```python
from build123d import *

# Parameters (mm, degrees)
SKETCH2_W                        = 127
SKETCH2_H                        = 127
HOUSING_DEPTH                    = 39.5
SKETCH3_R                        = 19.05
CUT_EXTRUDE1_DEPTH               = 40.5
SKETCH4_OUTSIDE_W                = 165.78
SKETCH4_OUTSIDE_H                = 165.78
SKETCH4_OUTSIDE_R                = 45.974
CUT_EXTRUDE2_DEPTH               = 4.698
MOUNTING_POCKETS_DEPTH           = 24.384
ENG_METRIC_SLOT_VERTICAL_REACH   = 129
ENG_METRIC_SLOT_HORIZONTAL_DEPTH = 40.5
FILLET3_R                        = 0.508
F_10_32_TAPPED_HOLE1_D           = 4.0386
F_10_32_TAPPED_HOLE1_DEPTH       = 12.02944
F_10_32_TAPPED_HOLE1_TIP         = 1.213317848
SKETCH219_R                      = 53.086
EXTRUDE2_DEPTH                   = 10.414
SKETCH222_R                      = 53.086
SKETCH222_R_2                    = 46.99
CUT_EXTRUDE6_DEPTH               = 6.35
LPATTERN14_COUNT                 = 3
LPATTERN14_PITCH                 = 25.4
LPATTERN14_COUNT_DIR2            = 3
LPATTERN14_PITCH_DIR2            = 25.4
M6X1_0_TAPPED_HOLE1_D            = 5
M6X1_0_TAPPED_HOLE1_DEPTH        = 8
M6X1_0_TAPPED_HOLE1_CBORE_D      = 6
M6X1_0_TAPPED_HOLE1_CBORE_DEPTH  = 6
M6X1_0_TAPPED_HOLE1_TIP          = 1.502151548
SKETCH234_W                      = 34.802
SKETCH234_H                      = 127
CUT_EXTRUDE8_DEPTH               = 128


with BuildPart() as part:
    # Sketch2 → HOUSING (new body)
    with BuildSketch(Plane.XY):
        Rectangle(SKETCH2_W, SKETCH2_H)
    extrude(amount=HOUSING_DEPTH)

    # Sketch3 → Cut-Extrude1 (cut, through all)
    with BuildSketch(Plane.XY.offset(39.5)):
        Circle(SKETCH3_R)
    extrude(amount=-CUT_EXTRUDE1_DEPTH, mode=Mode.SUBTRACT)

    # Sketch4 outside → Cut-Extrude2 (cut)
    with BuildSketch(Plane.XY.offset(39.5)):
        Rectangle(SKETCH4_OUTSIDE_W, SKETCH4_OUTSIDE_H)
        Circle(SKETCH4_OUTSIDE_R, mode=Mode.SUBTRACT)
    extrude(amount=-CUT_EXTRUDE2_DEPTH, mode=Mode.SUBTRACT)

    # Sketch8 → MOUNTING POCKETS (cut)
    with BuildSketch(Plane.XY.offset(34.802)):
        with BuildLine():
            Line((3.048, -63.5), (3.048, -57.528018122))
            ThreePointArc((3.048, -57.528018122), (4.194729662, -53.888172274), (7.220748912, -51.562946647))
            Line((7.220748912, -51.562946647), (45.320748912, -37.656446647))
            ThreePointArc((45.320748912, -37.656446647), (51.137845848, -38.418247784), (53.848, -43.621518122))
            Line((53.848, -43.621518122), (53.848, -63.5))
            Line((53.848, -63.5), (3.048, -63.5))
        make_face()
        with BuildLine():
            Line((3.048, 63.5), (53.848, 63.5))
            Line((53.848, 63.5), (53.848, 43.621518122))
            ThreePointArc((53.848, 43.621518122), (51.137845848, 38.418247784), (45.320748912, 37.656446647))
            Line((45.320748912, 37.656446647), (7.220748912, 51.562946647))
            ThreePointArc((7.220748912, 51.562946647), (4.194729662, 53.888172274), (3.048, 57.528018122))
            Line((3.048, 57.528018122), (3.048, 63.5))
        make_face()
    extrude(amount=-MOUNTING_POCKETS_DEPTH, mode=Mode.SUBTRACT)

    # Sketch21 → ENG_METRIC SLOT VERTICAL (cut, up to next)
    with BuildSketch(Plane(origin=(63.5, -23.646142673, 1.166551585), x_dir=(0, 0, -1), z_dir=(1, 0, 0)), mode=Mode.PRIVATE) as eng_metric_slot_vertical_sk1:
        with BuildLine():
            Line((-20.641506099, 75.242113831), (-21.041506099, 76.042113831))
            ThreePointArc((-21.041506099, 76.042113831), (-25.829419573, 77.63808499), (-27.425390732, 72.850171515))
            Line((-27.425390732, 72.850171515), (-27.025390732, 72.050171515))
            ThreePointArc((-27.025390732, 72.050171515), (-22.237477257, 70.454200357), (-20.641506099, 75.242113831))
        make_face()
    eng_metric_slot_vertical_tool1 = extrude(eng_metric_slot_vertical_sk1.sketch, amount=-ENG_METRIC_SLOT_VERTICAL_REACH, mode=Mode.PRIVATE) & part.part
    add(eng_metric_slot_vertical_tool1.solids().sort_by_distance((63.5, 50.4, 25.2))[0], mode=Mode.SUBTRACT)
    # Sketch21 → ENG_METRIC SLOT VERTICAL (cut, up to next)
    with BuildSketch(Plane(origin=(63.5, -23.646142673, 1.166551585), x_dir=(0, 0, -1), z_dir=(1, 0, 0)), mode=Mode.PRIVATE) as eng_metric_slot_vertical_sk2:
        with BuildLine():
            Line((-27.025390732, -24.757886169), (-27.425390732, -25.557886169))
            ThreePointArc((-27.425390732, -25.557886169), (-25.829419573, -30.345799643), (-21.041506099, -28.749828485))
            Line((-21.041506099, -28.749828485), (-20.641506099, -27.949828485))
            ThreePointArc((-20.641506099, -27.949828485), (-22.237477257, -23.16191501), (-27.025390732, -24.757886169))
        make_face()
    eng_metric_slot_vertical_tool2 = extrude(eng_metric_slot_vertical_sk2.sketch, amount=-ENG_METRIC_SLOT_VERTICAL_REACH, mode=Mode.PRIVATE) & part.part
    add(eng_metric_slot_vertical_tool2.solids().sort_by_distance((63.5, -50.4, 25.2))[0], mode=Mode.SUBTRACT)

    # Sketch212 → ENG_METRIC SLOT HORIZONTAL (cut, through all)
    with BuildSketch(Plane(origin=(34.062086582, -104.655987826, 0), x_dir=(-1, 0, 0), z_dir=(0, 0, -1))):
        with BuildLine():
            Line((12.254028899, 156.251958985), (11.854028899, 157.051958985))
            ThreePointArc((11.854028899, 157.051958985), (7.066115424, 158.647930143), (5.470144266, 153.860016668))
            Line((5.470144266, 153.860016668), (5.870144266, 153.060016668))
            ThreePointArc((5.870144266, 153.060016668), (10.658057741, 151.46404551), (12.254028899, 156.251958985))
        make_face()
        with BuildLine():
            Line((5.870144266, 56.251958985), (5.470144266, 55.451958985))
            ThreePointArc((5.470144266, 55.451958985), (7.066115424, 50.66404551), (11.854028899, 52.260016668))
            Line((11.854028899, 52.260016668), (12.254028899, 53.060016668))
            ThreePointArc((12.254028899, 53.060016668), (10.658057741, 57.847930143), (5.870144266, 56.251958985))
        make_face()
    extrude(amount=-ENG_METRIC_SLOT_HORIZONTAL_DEPTH, mode=Mode.SUBTRACT)

    # Fillet3
    fillet3_edges = [part.edges().sort_by_distance(p)[0] for p in [
        (3.048, -60.514009061, 10.418),
        (4.194729662, -53.888172274, 10.418),
        (26.270748912, -44.609696647, 10.418),
        (51.137845848, -38.418247784, 10.418),
        (53.848, -53.560759061, 10.418),
        (51.137845848, 38.418247784, 10.418),
        (26.270748912, 44.609696647, 10.418),
        (4.194729662, 53.888172274, 10.418),
        (3.048, 60.514009061, 10.418),
        (53.848, 53.560759061, 10.418),
    ]]
    fillet(fillet3_edges, radius=FILLET3_R)

    # #10-32 Tapped Hole1
    with Locations(Plane.XY.offset(39.5)):
        with Locations((26.9875, -26.9875), (26.9875, 26.9875), (-26.9875, 26.9875), (-26.9875, -26.9875)):
            Hole(F_10_32_TAPPED_HOLE1_D / 2, depth=F_10_32_TAPPED_HOLE1_DEPTH)
            with Locations((0, 0, -(F_10_32_TAPPED_HOLE1_DEPTH + F_10_32_TAPPED_HOLE1_TIP / 2))):  # 118° drill point
                Cone(0, F_10_32_TAPPED_HOLE1_D / 2, F_10_32_TAPPED_HOLE1_TIP, mode=Mode.SUBTRACT)

    # Sketch219 → Extrude2 (add)
    with BuildSketch(Plane.XY.offset(48.26)):
        Circle(SKETCH219_R)
    extrude(amount=-EXTRUDE2_DEPTH)

    # Sketch222 → Cut-Extrude6 (cut)
    with BuildSketch(Plane(origin=(0, 0, 37.846), x_dir=(-1, 0, 0), z_dir=(0, 0, -1))):
        Circle(SKETCH222_R)
        Circle(SKETCH222_R_2, mode=Mode.SUBTRACT)
    extrude(amount=-CUT_EXTRUDE6_DEPTH, mode=Mode.SUBTRACT)

    # Sketch230 → 1/4-20 Tapped Hole2 (revolve, cut)
    with BuildSketch(Plane(origin=(-25.4, 25.4, 48.26), x_dir=(0, -1, 0), z_dir=(1, 0, 0))):
        Polygon((0, 0), (0, 9.533816902), (2.5527, 8), (2.5527, 6), (3.175, 6), (3.175, 0), align=None)
    f_1_4_20_tapped_hole2 = revolve(axis=Axis((-25.4, 25.4, 54.61), (0, 0, -1)), mode=Mode.SUBTRACT)

    # LPattern14: 1_4-20 Tapped Hole2 3 × 3
    with Locations(*[(i * LPATTERN14_PITCH, -j * LPATTERN14_PITCH_DIR2, 0) for i in range(LPATTERN14_COUNT) for j in range(LPATTERN14_COUNT_DIR2) if (i, j) != (0, 0)]):
        add(f_1_4_20_tapped_hole2, mode=Mode.SUBTRACT)

    # M6x1.0 Tapped Hole1
    with Locations(Plane.XY.offset(48.26)):
        with Locations((-25, 25)):
            CounterBoreHole(M6X1_0_TAPPED_HOLE1_D / 2, M6X1_0_TAPPED_HOLE1_CBORE_D / 2, M6X1_0_TAPPED_HOLE1_CBORE_DEPTH, depth=M6X1_0_TAPPED_HOLE1_DEPTH)
            with Locations((0, 0, -(M6X1_0_TAPPED_HOLE1_DEPTH + M6X1_0_TAPPED_HOLE1_TIP / 2))):  # 118° drill point
                Cone(0, M6X1_0_TAPPED_HOLE1_D / 2, M6X1_0_TAPPED_HOLE1_TIP, mode=Mode.SUBTRACT)

    # Sketch234 → Cut-Extrude8 (cut, through all)
    with BuildSketch(Plane.ZY.offset(63.5)):
        with Locations((17.401, 0)):
            Rectangle(SKETCH234_W, SKETCH234_H)
    extrude(amount=-CUT_EXTRUDE8_DEPTH, mode=Mode.SUBTRACT)


solid = part.part
```
Verification items for the finished model (mm, model axes). A direction names the side the tool comes from. Coordinates: 2 decimals unless noted, no trailing zeros. Loops run counter-clockwise (first coordinate to the right, second up) from the corner with the lowest first, then second, coordinate; pieces in that order, holes last. Notation, with made-up numbers: (24, 60) - (41, 60) arc R32 ccw to (41, 98) - close; hole circle Ø2 at (10.25, -28). An arc over 180 degrees is marked (long way). Answer as a JSON object with one key per item and string values.
(1) Cross-section at B-B, the plane y = -36.5. Record the boundary of the cut face in (x, z).
Response:
{"outline": "(-38.55, 44.2) - (-29.59, 44.2) - (-29.59, 37.85) - (-27.95, 37.85) - (-27.95, 34.8) - (27.95, 34.8) - (27.95, 37.85) - (29.59, 37.85) - (29.59, 44.2) - (38.55, 44.2) - (38.55, 48.26) - (-38.55, 48.26) - close"}
(2) Scan lines: line 1 along Y through (x, z) = (0, 41.05); line 2 along Y through (x, z) = (25.4, 44.1) (3 decimals); line 3 along Z through (x, y) = (2, 27.5). Record each from-to range of solid material in increasing order.
Response:
{"line 1": "y = -46.99 to -27.95, -22.85 to -2.55, 2.55 to 22.85, 27.95 to 46.99", "line 2": "y = -39.534 to -28.575, -22.225 to -3.175, 3.175 to 22.225, 28.575 to 39.534", "line 3": "z = 34.8 to 42.26"}
(3) Cross-section at C-C, the plane x = -40. Record the boundary of the cut face in (y, z).
Response:
{"outline": "(-34.9, 44.2) - (-24.66, 44.2) - (-24.66, 37.85) - (-22.66, 37.85) - (-22.66, 34.8) - (22.66, 34.8) - (22.66, 37.85) - (24.66, 37.85) - (24.66, 44.2) - (34.9, 44.2) - (34.9, 48.26) - (-34.9, 48.26) - close"}
(4) Cross-section at A-A, the plane z = 45.5. Count the separate pieces of the cut face and the enclosed holes in it, then the cut area to 3 significant figures.
Response:
{"separate pieces": "1", "enclosed holes": "9", "area": "8,570 mm²"}
(5) Cross-section at D-D, the plane z = 36.5. Record the boundary of the cut face in (x, y), then the cut area to 3 significant figures.
Response:
{"outline": "circle Ø91.95 at (0, 0); hole circle Ø4.04 at (-26.99, -26.99); hole circle Ø4.04 at (-26.99, 26.99); hole circle Ø38.1 at (0, 0); hole circle Ø4.04 at (26.99, -26.99); hole circle Ø4.04 at (26.99, 26.99)", "area": "5,450 mm²"}
(6) Mould release check, pull along Y, two halves, no side actions. Record for faces 3 (the cylindrical face through (-28.077, -27.107, 45.302)), 4 (the cylindrical face through (24.715, 38.765, 36.345)), 5 (the flat face through (31, -35, 37.846)): pulls with the +Y half, pulls with the -Y half, needs draft (parallel to the pull), parting line crosses it, or undercut.
Response:
{"face 3": "undercut", "face 4": "parting line crosses it", "face 5": "needs draft"}
(7) Access from +Z, -Z, +X, -X, +Y, -Y to the whole of each face (thin tool, end or side, straight path). Record for faces 1 (the cylindrical face through (-26.725, -24.985, 36.303)), 2 (the cylindrical face through (22.25, 0.41, 45.3)).
Response:
{"face 1": "-Z", "face 2": "+Z"}
(8) Go/stop test with flat-tipped pins: pin 1 Ø1.9 at (x, y) = (26.5, -1) entering from +Z; pin 2 Ø4 at (x, z) = (-26, 39.5) entering from +Y; pin 3 Ø6 at (x, z) = (-20.5, 47) entering from +Y. Record where each tip stops, or that it passes through.
Response:
{"pin 1": "stops at z = 40.19", "pin 2": "stops at y = 40.4", "pin 3": "stops at y = 50.12"}
